Source: CAD feature listing. Evaluate the final solid. Frame: model axes, mm. Give positions to 0.01 mm unless a question says otherwise; leave off trailing zeros. Order: outer loops, then holes, each group sorted by start corner. A loop starts at its lowest first (then second) coordinate and runs counter-clockwise, first axis right, second up. Notation, with made-up numbers: M -27,22.25 L -2,22.25 A14 cw -2,38.25 Z; hole C 64.25,-6 d5. An arc over 180 degrees is marked long. Use CSV: the item, a comma, the result in double quotes. Start each with the question number.
Item 1: Section query A-A on x = 5.5. Return loops of the section in (y, z).
Item 2: Section query C-C on y = -12. Return loops of the section in (x, z).
Item 3: Ray query, probe 1 along Y at (x, z) = (0, 0.75); probe 2 along Y at (x, z) = (-8.5, 1.4); probe 3 along Y at (x, z) = (-8, 0.65). Return the intervals inside material, ascending. Write a range as from..to.
Item 4: Section query D-D on y = 10. Return loops of the section in (x, z).
Item 5: First-contact query: pin 1 (1.7 mm diameter, centred on x = 0, y = -18.415, fed in from -Z). Flat tip, straight axial feed; report the tip coordinate or a pass-through.
Item 6: Section query B-B on z = 1.05. Return loops of the section in (x, y) (1 decimal), and give its area (3 significant figures).
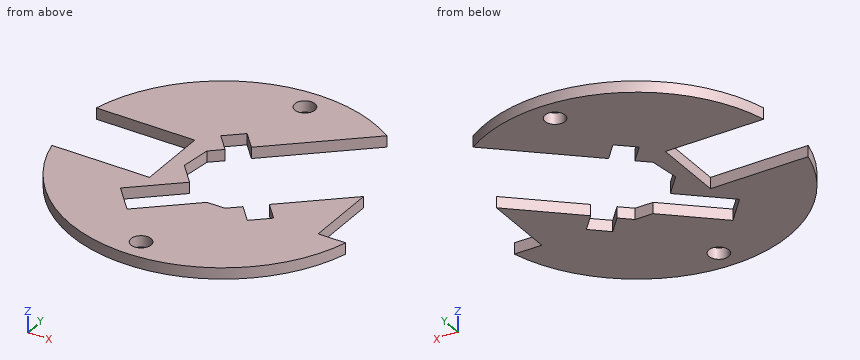
from build123d import *

# Parameters (mm, degrees)
SKETCH1_R           = 1.4224
BOSS_EXTRUDE1_DEPTH = 1.5875
CUT_EXTRUDE3_DEPTH  = 31.574112518
CUT_EXTRUDE4_DEPTH  = 31.574112518


with BuildPart() as part:
    # Sketch1 → Boss-Extrude1 (new body)
    with BuildSketch(Plane.XY):
        with BuildLine():
            Line((-5.027565338, -0.720652536), (-4.515281158, 3.5306))
            Line((-4.515281158, 3.5306), (-2.860140414, 4.994714494))
            Line((-2.860140414, 4.994714494), (-4.980602482, 7.391837931))
            Line((-4.980602482, 7.391837931), (-2.583479045, 9.5123))
            Line((-2.583479045, 9.5123), (-0.463016976, 7.115176563))
            Line((-0.463016976, 7.115176563), (11.876076152, 18.030166811))
            ThreePointArc((11.876076152, 18.030166811), (-16.886200405, -13.453041882), (20.228041911, 7.546815251))
            Line((20.228041911, 7.546815251), (8.405899773, -2.910887338))
            Line((8.405899773, -2.910887338), (10.526361842, -5.308010776))
            Line((10.526361842, -5.308010776), (8.129238404, -7.428472845))
            Line((8.129238404, -7.428472845), (6.008776335, -5.031349407))
            Line((6.008776335, -5.031349407), (4.353635591, -6.495463901))
            Line((4.353635591, -6.495463901), (1.815981702, -6.489359631))
            Line((1.815981702, -6.489359631), (-5.455454601, -12.9215711))
            Line((-5.455454601, -12.9215711), (-8.720293025, -9.230761998))
            Line((-8.720293025, -9.230761998), (-2.425370717, -3.662361234))
            Line((-2.425370717, -3.662361234), (-5.027565338, -0.720652536))
        make_face()
        with Locations((0, 18.415)):
            Circle(SKETCH1_R, mode=Mode.SUBTRACT)
        with Locations((0, -18.415)):
            Circle(SKETCH1_R, mode=Mode.SUBTRACT)
    extrude(amount=BOSS_EXTRUDE1_DEPTH)

    # Sketch2 → Cut-Extrude3 (cut, through all)
    with BuildSketch(Plane.XY.offset(1.5875)):
        with BuildLine():
            Line((-7.084965338, 4.8768), (-21.031997569, 4.8768))
            ThreePointArc((-21.031997569, 4.8768), (-21.588987692, -0.209070373), (-20.933606898, -5.2832))
            Line((-20.933606898, -5.2832), (-7.084965338, -5.2832))
            Line((-7.084965338, -5.2832), (-7.084965338, 4.8768))
        make_face()
    extrude(amount=-CUT_EXTRUDE3_DEPTH, mode=Mode.SUBTRACT)

    # Sketch3 → Cut-Extrude4 (cut, through all)
    with BuildSketch(Plane(origin=(0, 0, 0), x_dir=(-1, 0, 0), z_dir=(0, 0, -1))):
        with BuildLine():
            Line((-20.871224203, -5.5245), (-16.984058744, -5.5245))
            Line((-16.984058744, -5.5245), (-16.984058744, 4.677232838))
            Line((-16.984058744, 4.677232838), (-20.228041911, 7.546815251))
            ThreePointArc((-20.228041911, 7.546815251), (-21.563910577, 1.061065789), (-20.871224203, -5.5245))
        make_face()
    extrude(amount=-CUT_EXTRUDE4_DEPTH, mode=Mode.SUBTRACT)


solid = part.part
Verdict:
1,outline,"M -20.88,0 L -5.48,0 L -5.48,1.59 L -20.88,1.59 Z; M 12.39,0 L 20.88,0 L 20.88,1.59 L 12.39,1.59 Z"
2,outline,"M -17.95,0 L -6.27,0 L -6.27,1.59 L -17.95,1.59 Z; M -4.41,0 L 17.95,0 L 17.95,1.59 L -4.41,1.59 Z"
3,probe 1,"-21.59..-19.84, -16.99..-8.1, 7.52..16.99, 19.84..21.59"
3,probe 2,"-19.85..-9.48, -9.04..-5.28, 4.88..19.85"
3,probe 3,"-20.05..-10.05, -8.59..-5.28, 4.88..20.05"
4,outline,"M -19.13,0 L 2.8,0 L 2.8,1.59 L -19.13,1.59 Z"
5,pin 1,"through"
6,outline,"M -21,4.9 L -7.1,4.9 L -7.1,-5.3 L -20.9,-5.3 A21.6 ccw 20.9,-5.5 L 17,-5.5 L 17,4.7 L 8.4,-2.9 L 10.5,-5.3 L 8.1,-7.4 L 6,-5 L 4.4,-6.5 L 1.8,-6.5 L -5.5,-12.9 L -8.7,-9.2 L -2.4,-3.7 L -5,-0.7 L -4.5,3.5 L -2.9,5 L -5,7.4 L -2.6,9.5 L -0.5,7.1 L 11.9,18 A21.6 ccw Z; hole C 0,-18.4 d2.8; hole C 0,18.4 d2.8"
6,area,"861 mm2"
